Could you check a few things on this model? Use its own coordinates, in mm. A direction names the side the tool comes from. Round coordinates to 2 decimals unless told otherwise and drop trailing zeros. Loops run counter-clockwise (first coordinate to the right, second up) from the corner with the lowest first, then second, coordinate; pieces in that order, holes last. Notation, with made-up numbers: M -6,13.25 L -2,13.25 A12 ccw -2,28.25 Z; hole C -15.5,71 d11. An arc over 180 degrees is marked long. Answer in a Markdown table with one row per item.
```python
from build123d import *

# Parameters (mm, degrees)
F0_W     = 200
F0_H     = 337
F1_DEPTH = 18.1
F2_W     = 25
F2_H     = 18.6
F2_W_2   = 150
F3_DEPTH = 10
F5_DEPTH = 25
F6_W     = 7
F6_H     = 209.4
F7_DEPTH = 10
F8_W     = 7
F8_H     = 109
F9_DEPTH = 10


with BuildPart() as f1:
    # F0 (on Top) → F1 (new body)
    with BuildSketch(Plane.XY):
        Rectangle(F0_W, F0_H)
    extrude(amount=F1_DEPTH)

    # F2 (on face) → F3 (cut)
    with BuildSketch(Plane.XY.offset(18.1)):
        with Locations((-87.5, -50.2)):
            Rectangle(F2_W, F2_H)
        with Locations((-62.5, -50.2)):
            Rectangle(F2_W, F2_H)
        with Locations((25, -50.2)):
            Rectangle(F2_W_2, F2_H)
        with Locations((112.5, -50.2)):
            Rectangle(F2_W, F2_H)
        with Locations((137.5, -50.2)):
            Rectangle(F2_W, F2_H)
    extrude(amount=-F3_DEPTH, mode=Mode.SUBTRACT)

    # F4 (on face) → F5 (cut)
    with BuildSketch(Plane.XY.offset(8.1)):
        with BuildLine():
            Line((-52.5, -50.2), (-50, -50.2))
            Line((-50, -50.2), (-47.5, -50.2))
            ThreePointArc((-47.5, -50.2), (-50, -47.7), (-52.5, -50.2))
        make_face()
        with BuildLine():
            Line((-47.5, -50.2), (-50, -50.2))
            Line((-50, -50.2), (-52.5, -50.2))
            ThreePointArc((-52.5, -50.2), (-50, -52.7), (-47.5, -50.2))
        make_face()
        with BuildLine():
            ThreePointArc((52.5, -50.2), (50, -47.7), (47.5, -50.2))
            Line((47.5, -50.2), (50, -50.2))
            Line((50, -50.2), (52.5, -50.2))
        make_face()
        with BuildLine():
            Line((50, -50.2), (47.5, -50.2))
            ThreePointArc((47.5, -50.2), (50, -52.7), (52.5, -50.2))
            Line((52.5, -50.2), (50, -50.2))
        make_face()
    extrude(amount=-F5_DEPTH, mode=Mode.SUBTRACT)

    # F6 (on face) → F7 (cut)
    with BuildSketch(Plane.XY.offset(18.1)):
        with Locations((-91.5, 63.8)):
            Rectangle(F6_W, F6_H)
    extrude(amount=-F7_DEPTH, mode=Mode.SUBTRACT)

    # F8 (on face) → F9 (cut)
    with BuildSketch(Plane.XY.offset(18.1)):
        with Locations((-91.5, -114)):
            Rectangle(F8_W, F8_H)
    extrude(amount=-F9_DEPTH, mode=Mode.SUBTRACT)


solid = f1.part
```
1) Will this pin go through, and if not, where does the flat tip stop? P1, Ø3, axis at x = -50, y = -50.2, coming from the -Z side.
Computed:
| item | result |
|---|---|
| P1 | passes through |
2) I want a section at C-C, the plane y = -25. Please give me the cut outline in (x, z), plus the area to 3 significant figures.
Computed:
| item | result |
|---|---|
| outline | M -100,0 L 100,0 L 100,18.1 L -88,18.1 L -88,8.1 L -95,8.1 L -95,18.1 L -100,18.1 Z |
| area | 3,550 mm² |
3) I need wall thicknesses on line 1 (Y direction, x = 50, z = 5.75); line 2 (Y direction, x = 87, z = 10); line 3 (X direction, y = -99, z = 14.25). Which ranges of each line are inside material? Lowest first, please.
Computed:
| item | result |
|---|---|
| line 1 | y = -168.5 to -52.7, -47.7 to 168.5 |
| line 2 | y = -168.5 to -59.5, -40.9 to 168.5 |
| line 3 | x = -100 to -95, -88 to 100 |
4) I want a section at A-A, the plane z = 15. Please give me the cut outline in (x, y).
Computed:
| item | result |
|---|---|
| outline | M -100,-168.5 L -95,-168.5 L -95,-59.5 L -100,-59.5 Z; M -100,-40.9 L -95,-40.9 L -95,168.5 L -100,168.5 Z; M -88,-168.5 L 100,-168.5 L 100,-59.5 L -88,-59.5 Z; M -88,-40.9 L 100,-40.9 L 100,168.5 L -88,168.5 Z |
5) Which directions (+Z, -Z, +X, -X, +Y, -Y) give clear straight access to the entire face, cutting with the end or side of a thin tool? Please do faces 1 (the face through (5, -59.5, 13)), 2 (the face through (-95, 62, 13)), 3 (the face through (-1, -168.5, 9)).
Computed:
| item | result |
|---|---|
| face 1 | +Z, +X, -X |
| face 2 | +Z, +Y, -Y |
| face 3 | +Z, -Z, +X, -X, -Y |
6) If we mould it in two halves opening along X, with no side actions, what happens to faces 4 (the face through (-88, 62, 13)), 5 (the face through (-100, -2, 9)), 6 (the face through (-1, 168.5, 9)), 7 (the face through (-45, -49, 8.1))? For each: released by +X, released by -X, zero draft, split by the parting line, or undercut.
Computed:
| item | result |
|---|---|
| face 4 | undercut |
| face 5 | released by -X |
| face 6 | zero draft |
| face 7 | undercut |
7) I want a section at B-B, the plane x = -76. Please give me the cut outline in (y, z), plus the area to 3 significant figures.
Computed:
| item | result |
|---|---|
| outline | M -168.5,0 L 168.5,0 L 168.5,18.1 L -40.9,18.1 L -40.9,8.1 L -59.5,8.1 L -59.5,18.1 L -168.5,18.1 Z |
| area | 5,910 mm² |
